Design review of the part built by this model. Coordinates are the model's own, in mm. A direction names the side the tool comes from. Coordinates: 2 decimals unless noted, no trailing zeros. Order: outer loops, then holes, each group sorted by start corner. A loop starts at its lowest first (then second) coordinate and runs counter-clockwise, first axis right, second up. Notation, with made-up numbers: M 49,58 L 88,58 A19 ccw 88,78 Z; hole C 78,58.5 d7. An arc over 180 degrees is marked long. Use CSV: the item, a comma, the result in double quotes.
Autodesk Inventor part; units mm, degrees
ref_plane "作業平面1" through (230, 0, 0) normal (1, 0, 0) x (0, 1, 0)
ref_plane "作業平面2" through (589, 0, 0) normal (-1, 0, 0) x (0, 0, 1)
ref_plane "作業平面3" through (230, 0, 0) normal (1, 0, 0) x (0, 1, 0)
sketch "スケッチ1" plane through (0, 0, 0) normal (1, 0, 0) x (0, 1, 0)
  line L0 (10, 175) -> (0, 175)
  line L1 (0, 175) -> (0, -175)
  line L2 (0, -175) -> (10, -175)
  line L3 (10, -175) -> (10, 175)
  point P0 (0, 0)
  dimension "d0" = 350
  dimension "d1" = 10
extrude "押し出し1" add sketch "スケッチ1" along normal mid plane 1350
sketch "スケッチ2" plane through (675, 0, 0) normal (1, 0, 0) x (0, 0, -1)
  line L0 (-15.1924, 200) -> (-275, 50)
  line L1 (-275, 50) -> (-275, -50)
  line L2 (-275, -50) -> (325, -50)
  line L3 (325, -50) -> (325, 200)
  line L4 (-175, 0) -> (175, 0)
  line L5 (-175, 10) -> (-175, 0)
  line L6 (175, 0) -> (175, 10)
  line L7 (175, 10) -> (-175, 10)
  line L8 (-15.1924, 200) -> (325, 200)
  point P0 (0, 0)
  dimension "d4" = 50
  dimension "d5" = 30
  dimension "d6" = 250
  dimension "d7" = 600
  dimension "d8" = 100
  dimension "d9" = 100
extrude "押し出し3" add sketch "スケッチ2" along normal blind 10 contours L8 L3 L2 L1 L0 | L5 L7 L6 L4
ref_plane "作業平面1" through (230, 0, 0) normal (1, 0, 0) x (0, 1, 0)
ref_plane "作業平面2" through (589, 0, 0) normal (-1, 0, 0) x (0, 0, 1)
ref_plane "作業平面3" through (230, 0, 0) normal (1, 0, 0) x (0, 1, 0)
mirror "ミラー3" about plane through (589, 0, 0) normal (-1, 0, 0) of "押し出し3"
sketch "スケッチ4" plane through (230, 0, 0) normal (1, 0, 0) x (0, 1, 0)
  line L0 (70, 245) -> (-30, 245)
  line L1 (-30, 245) -> (-30, -375)
  line L2 (-30, -375) -> (250, -375)
  line L3 (250, -375) -> (250, -66.7691)
  line L4 (250, -66.7691) -> (70, 245)
  line L5 (0, -505) -> (0, 405)
  line L6 (50, 275) -> (-50, 275)
  line L7 (-50, 275) -> (-50, -325)
  line L8 (-50, -325) -> (200, -325)
  line L9 (200, -325) -> (200, 15.1924)
  point P0 (0, 0)
  dimension "d26" = 30
  dimension "d27" = 20
  dimension "d28" = 50
  dimension "d29" = 30
  dimension "d30" = 100
  dimension "d44" = 50
extrude "押し出し5" add sketch "スケッチ4" along normal blind 10 contours L4 L3 L2 L5 L0 | L5 L8 L1 L0 | L5 L2 L1 L8
sketch "スケッチ5" plane through (675, 0, 0) normal (-1, 0, 0) x (0, 0, 1)
  arc A0 (-243.2616, 197.5471) -> (-45, 20) centre (-11.1877, 257.2271) ccw
  line L0 (175, 10) -> (-175, 10)
  line L1 (-175, 10) -> (-175, 0)
  line L2 (-175, 10) -> (-243.2616, 197.5471)
  arc A1 (-243.2616, 197.5471) -> (-45, 20) centre (-61.7359, 200.7814) ccw
  point P0 (0, 0)
  dimension "d36" = 10
  dimension "d37" = 130
  dimension "d42" = 110
extrude "押し出し6" add sketch "スケッチ5" along normal up to next contours A0 L2 A1 | A0 A1 L2
fillet "フィレット1" radius 2 2 edges at (589, 197.5471, -243.2616) (589, 20, -45)
mirror "ミラー6" about plane through (0, 0, 0) normal (1, 0, 0) of "押し出し5", "押し出し3", "ミラー3", "押し出し6", "フィレット1"
properties part number "F-wing" material "PAEK 樹脂"
(1) Add section A-A on y = 120. Give the number of separate pieces and of enclosed holes in the cut face, and give its area (3 significant figures).
The answers:
separate pieces,"4"
enclosed holes,"0"
area,"35,600 mm2"
(2) Wall thickness on probe 1 along X at (y, z) = (182.5, -233); probe 2 along X at (y, z) = (-32, -194.5); probe 3 along Y at (x, z) = (-287.5, 106): over which ranges is each line inside the solid? List them lowest first.
The answers:
probe 1,"x = -685 to -675, -503 to -493, -240 to -230, 230 to 240, 493 to 503, 675 to 685"
probe 2,"x = -685 to -675, -503 to -493, 493 to 503, 675 to 685"
probe 3,"y = 0 to 10"
(3) The part is to be moulded in two halves that separate along X. For faces 1 (the face through (-234.93, 158.74, 91.3)), 2 (the face through (-240, 112, -130)), 3 (the face through (-685, 77, -29)), say which applies: pulls with the +X half, pulls with the -X half, needs draft (parallel to the pull), parting line crosses it, or undercut.
The answers:
face 1,"needs draft"
face 2,"undercut"
face 3,"pulls with the -X half"
(4) Clearance check with flat-ended pins moving along their axes: P1, Ø12, axis at x = -186, z = -137.5, coming from the +Y side; P2, Ø11, axis at x = 497, y = 52.5, coming from the -Z side; P3, Ø11, axis at x = -29.5, y = 2.5, coming from the +Z side. State where each tip first meets the part, or that it passes through.
The answers:
P1,"stops at y = 10"
P2,"stops at z = -325"
P3,"stops at z = 175"
(5) Add section B-B on z = -304. State the section outline as (x, y) points, and give its area (3 significant figures).
The answers:
outline,"M -685,-50 L -675,-50 L -675,200 L -685,200 Z; M -503,-50 L -493,-50 L -493,200 L -503,200 Z; M -240,-30 L -230,-30 L -230,250 L -240,250 Z; M 230,-30 L 240,-30 L 240,250 L 230,250 Z; M 493,-50 L 503,-50 L 503,200 L 493,200 Z; M 675,-50 L 685,-50 L 685,200 L 675,200 Z"
area,"15,600 mm2"
(6) Add section D-D on x = 76. State the section outline as (y, z) points, and give its area (3 significant figures).
The answers:
outline,"M 0,-175 L 10,-175 L 10,175 L 0,175 Z"
area,"3,500 mm2"
(7) For faces 4 (the face through (-590, 0, 2)), 5 (the face through (-368, 10, -2)), 6 (the face through (-590, 10, -2)), list the 3-axis set-ups (+Z, -Z, +X, -X, +Y, -Y) from which the entire face can be reached by the end or side of a thin tool; tool diameter is ignored.
The answers:
face 4,"+Z, -Z, -Y"
face 5,"+Z, -Z, +Y"
face 6,"+Z, -Z"
